Autodesk Inventor part; units mm, degrees
ref_plane "YZ Plane" through (0, 0, 0) normal (1, 0, 0) x (0, 1, 0)
ref_plane "XZ Plane" through (0, 0, 0) normal (0, 1, 0) x (-1, 0, 0)
ref_plane "XY Plane" through (0, 0, 0) normal (0, 0, 1) x (1, 0, 0)
sketch "Sketch1" plane through (0, 0, 0) normal (0, 1, 0) x (-1, 0, 0)
  line L0 (5, -12.5) -> (-5, -12.5)
  line L1 (-5, -12.5) -> (-5, 12.5)
  line L2 (-5, 12.5) -> (5, 12.5)
  line L3 (5, 12.5) -> (5, -12.5)
  line L4 (5, 0) -> (-5, 0)
  line L5 (0, -12.5) -> (0, 12.5)
  point P0 (0, 0)
  dimension "d1" = 10
  dimension "d2" = 25
extrude "Extrusion1" add sketch "Sketch1" along normal blind 10
sketch "Sketch2" plane through (-5, 0, 12.5) normal (0, 0, 1) x (1, 0, 0)
  line L0 (10, 0) -> (10, 10)
  line L1 (0, 0) -> (10, 0)
  line L2 (0, 0) -> (0, 10)
  line L3 (0, 10) -> (10, 10)
  line L4 (5, 10) -> (5, 0)
  line L5 (0.9, 9.1) -> (9.1, 9.1)
  line L6 (9.1, 9.1) -> (9.1, 0.9)
  line L7 (9.1, 0.9) -> (0.9, 0.9)
  line L8 (0.9, 0.9) -> (0.9, 9.1)
  line L9 (5, 9.1) -> (5, 0.9)
  line L10 (0, 5) -> (10, 5)
  line L11 (0.9, 5) -> (9.1, 5)
  line L12 (5, 9.1) -> (5, 0.9)
  point P0 (5, 5)
  point P1 (5, 5)
  dimension "d9" = 8.2
  dimension "d10" = 8.2
extrude "Extrusion2" cut sketch "Sketch2" against normal through all contours L10 L4 L5 L6 | L6 L7 L4 L10 | L7 L8 L10 L4 | L10 L8 L5 L4
sketch "Sketch5" plane through (0, 10, 0) normal (0, 1, 0) x (1, 0, 0)
  line L0 (-12.5, 5) -> (12.5, 5)
  line L1 (12.5, 5) -> (12.5, -5)
  line L2 (12.5, -5) -> (-12.5, -5)
  line L3 (-12.5, -5) -> (-12.5, 5)
  line L4 (-12.5, 0) -> (12.5, 0)
  line L5 (0, 5) -> (0, -5)
  point P0 (0, 0)
  dimension "d32" = 25
  dimension "d33" = 10
extrude "Extrusion4" add sketch "Sketch5" along normal blind 2
sketch "Sketch7" plane through (0, 12, 0) normal (0, 1, 0) x (1, 0, 0)
  line L0 (-12.5, 5) -> (-12.5, -5)
  line L1 (-12.5, 0) -> (12.5, 0)
  line L2 (12.5, -5) -> (12.5, 5)
  point P0 (0, 0)
  point P1 (-9.5, 0)
  point P2 (9.5, 0)
  dimension "d53" = 19
  dimension "d54" = 9.5
hole "Hole3" at (9.5, 12, 0) at (-9.5, 12, 0) direction (0, -1, 0) diameter 1.55 end through all
properties part number "Motor Mount"
Here's how the part is built. I have some questions about the finished solid (model axes, mm). A direction names the side the tool comes from. Coordinates: 2 decimals unless noted, no trailing zeros. Order: outer loops, then holes, each group sorted by start corner. A loop starts at its lowest first (then second) coordinate and runs counter-clockwise, first axis right, second up.
Item 1: If we section it at A-A, the plane z = 0: List the corners of the cut face in (x, y) for me (3 decimals).
Response values:
outline: (-12.5, 10) - (-10.275, 10) - (-10.275, 12) - (-12.5, 12) - close; (-8.725, 10) - (-5, 10) - (-5, 0) - (5, 0) - (5, 10) - (8.725, 10) - (8.725, 12) - (-8.725, 12) - close; (10.275, 10) - (12.5, 10) - (12.5, 12) - (10.275, 12) - close; hole (-4.1, 0.9) - (4.1, 0.9) - (4.1, 9.1) - (-4.1, 9.1) - close
Item 2: I need wall thicknesses on probe 1 along X at (y, z) = (10.55, 0) (3 decimals); probe 2 along X at (y, z) = (5.5, -2); probe 3 along Y at (x, z) = (-0.5, 3.25). Which ranges of each line are inside material? Lowest first, please.
Response values:
probe 1: x = -12.5 to -10.275, -8.725 to 8.725, 10.275 to 12.5
probe 2: x = -5 to -4.1, 4.1 to 5
probe 3: y = 0 to 0.9, 9.1 to 12
Item 3: If we section it at C-C, the plane y = 2.5: List the corners of the cut face in (x, z) for me.
Response values:
outline: (-5, -12.5) - (-4.1, -12.5) - (-4.1, 12.5) - (-5, 12.5) - close; (4.1, -12.5) - (5, -12.5) - (5, 12.5) - (4.1, 12.5) - close
Item 4: If we section it at D-D, the plane z = 6.75: List the corners of the cut face in (x, y) for me.
Response values:
outline: (-5, 0) - (5, 0) - (5, 10) - (-5, 10) - close; hole (-4.1, 0.9) - (4.1, 0.9) - (4.1, 9.1) - (-4.1, 9.1) - close
Item 5: Which directions (+Z, -Z, +X, -X, +Y, -Y) give clear straight access to the entire face, cutting with the end or side of a thin tool? Please do faces 1 (the face through (-8, 10, 0)), 2 (the face through (0, 11, 5)), 3 (the face through (8, 10, 0)), 4 (the face through (0, 10, -9)), 5 (the face through (0, 0.9, 0)).
Response values:
face 1: +Z, -Z, -X, -Y
face 2: +Z, +X, -X, +Y
face 3: +Z, -Z, +X, -Y
face 4: -Z, +X, -X, +Y
face 5: +Z, -Z
Item 6: If we section it at B-B, the plane x = 9.5: List the corners of the cut face in (y, z) for me (3 decimals), then the cut area to 3 significant figures.
Response values:
outline: (10, -5) - (12, -5) - (12, -0.775) - (10, -0.775) - close; (10, 0.775) - (12, 0.775) - (12, 5) - (10, 5) - close
area: 16.9 mm2
Item 7: Thinking about a two-plate mould opening in Z: for faces 6 (the face through (0, 10, 9)), 7 (the face through (0.1, 9.4, 12.5)), 8 (the face through (-10.27, 10.99, -0.1)), which applies, pulls with the +Z half, pulls with the -Z half, needs draft (parallel to the pull), parting line crosses it, or undercut?
Response values:
face 6: needs draft
face 7: pulls with the +Z half
face 8: undercut
Item 8: I'm going to push flat-ended pins straight in: pin 1 Ø2.5 at (y, z) = (6.5, -2.5) entering from +X; pin 2 Ø1.6 at (x, y) = (1.5, 11.5) entering from +Z; pin 3 Ø4 at (x, z) = (1, -9.5) entering from +Y. Where does each tip first touch, or does it pass through?
Response values:
pin 1: stops at x = 5
pin 2: stops at z = 5
pin 3: stops at y = 10
